Geometry: final body of the model. Coordinates: model frame, mm. Face numbers are marked on the shaded views. A direction names the side the tool comes from. Coordinates: 2 decimals unless noted, no trailing zeros. Write each loop counter-clockwise with the first axis right and the second up, starting at its lowest first coordinate (ties: lowest second). Pieces come first, ordered by that corner, then holes.
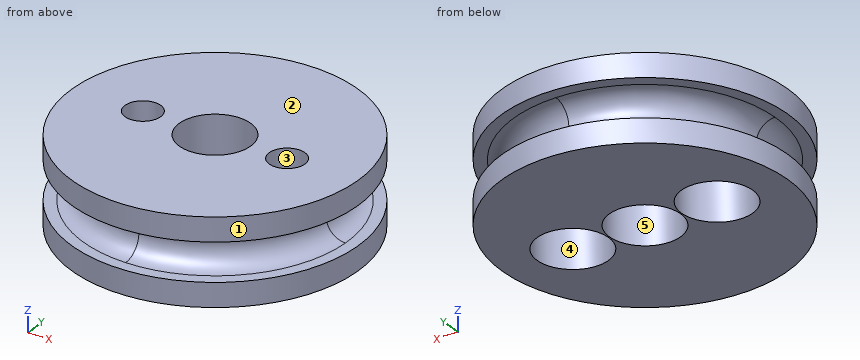
from build123d import *

# Parameters (mm, degrees)
SKETCH_1_R          = 12
EXTRUDE_1_DEPTH     = 2
SKETCH_2_R          = 11
EXTRUDE_2_DEPTH     = 3.2
SKETCH_3_R          = 12
EXTRUDE_3_DEPTH     = 2
SKETCH_4_R          = 3
CUT_EXTRUDE_1_DEPTH = 30
SKETCH_5_R          = 1.5
CUT_EXTRUDE_4_DEPTH = 19.434749795
SKETCH_3D_2_R       = 1.600287212
SKETCH_7_R          = 3
CUT_EXTRUDE_9_DEPTH = 4


with BuildPart() as part:
    # ｽｹｯﾁ1 → ﾎﾞｽ - 押し出し1 (new body)
    with BuildSketch(Plane.XY):
        Circle(SKETCH_1_R)
    extrude(amount=EXTRUDE_1_DEPTH)

    # ｽｹｯﾁ2 → ﾎﾞｽ - 押し出し2 (add)
    with BuildSketch(Plane.XY.offset(2)):
        Circle(SKETCH_2_R)
    extrude(amount=EXTRUDE_2_DEPTH)

    # ｽｹｯﾁ3 → ﾎﾞｽ - 押し出し3 (add)
    with BuildSketch(Plane.XY.offset(5.2)):
        Circle(SKETCH_3_R)
    extrude(amount=EXTRUDE_3_DEPTH)

    # ｽｹｯﾁ4 → ｶｯﾄ - 押し出し1 (cut)
    with BuildSketch(Plane(origin=(0, 0, 0), x_dir=(-1, 0, 0), z_dir=(0, 0, -1))):
        Circle(SKETCH_4_R)
    extrude(amount=-CUT_EXTRUDE_1_DEPTH, mode=Mode.SUBTRACT)

    # ｽｹｯﾁ5 → ｶｯﾄ - 押し出し4 (cut, through all)
    with BuildSketch(Plane(origin=(0, 0, 0), x_dir=(-1, 0, 0), z_dir=(0, 0, -1))):
        with Locations((-6.1, 0)):
            Circle(SKETCH_5_R)
        with Locations((6.1, 0)):
            Circle(SKETCH_5_R)
    extrude(amount=-CUT_EXTRUDE_4_DEPTH, mode=Mode.SUBTRACT)

    # ｶｯﾄ - ｽｲｰﾌﾟ2: sweep along a curve in space
    with BuildLine() as sweep_2_path:
        ThreePointArc((11, 0, 5.2), (7.778174593, 7.778174593, 5.2), (0, 11, 5.2))
        ThreePointArc((0, 11, 5.2), (-7.778174593, 7.778174593, 5.2), (-11, 0, 5.2))
        ThreePointArc((-11, 0, 5.2), (-7.778174593, -7.778174593, 5.2), (0, -11, 5.2))
        ThreePointArc((0, -11, 5.2), (7.778174593, -7.778174593, 5.2), (11, 0, 5.2))
    # Sketch 3D_2 → ｶｯﾄ - ｽｲｰﾌﾟ2 (sweep, cut)
    with BuildSketch(Plane(origin=(-11, 0, 5.2), x_dir=(0, 0, -1), z_dir=(0, -1, 0))):
        with Locations((1.600287212, 0)):
            Circle(SKETCH_3D_2_R)
    sweep(path=sweep_2_path.line, mode=Mode.SUBTRACT)

    # ｽｹｯﾁ7 → ｶｯﾄ - 押し出し9 (cut)
    with BuildSketch(Plane(origin=(0, 0, 0), x_dir=(-1, 0, 0), z_dir=(0, 0, -1))):
        with Locations((-6.1, 0)):
            Circle(SKETCH_7_R)
        with Locations((6.1, 0)):
            Circle(SKETCH_7_R)
    extrude(amount=-CUT_EXTRUDE_9_DEPTH, mode=Mode.SUBTRACT)


solid = part.part
Item 1: Section C-C, the plane z = 1.25. Output: boundary loops of the cut face in (x, y), plus the area to 3 significant figures.
Derived:
outline: circle Ø24 at (0, 0); hole circle Ø6 at (-6.1, 0); hole circle Ø6 at (0, 0); hole circle Ø6 at (6.1, 0)
area: 368 mm2
Item 2: Material intervals for probe 1 along Z at (x, y) = (-5.75, 10.5); probe 2 along X at (y, z) = (0.5, 3.5); probe 3 along X at (y, z) = (-0.5, 5.75), sorted ascending.
Derived:
probe 1: z = 0 to 2, 5.2 to 7.2
probe 2: x = -9.39 to -9.06, -3.14 to -2.96, 2.96 to 3.14, 9.06 to 9.39
probe 3: x = -11.99 to -7.51, -4.69 to -2.96, 2.96 to 4.69, 7.51 to 11.99
Item 3: Pull-direction query (Y, two-part tool) for the marked faces 1, 2 and 3; classes: released by +Y, released by -Y, zero draft, split by the parting line, or undercut.
Derived:
face 1: split by the parting line
face 2: zero draft
face 3: undercut
Item 4: Section A-A, the plane z = 6.5. Output: boundary loops of the cut face in (x, y).
Derived:
outline: circle Ø24 at (0, 0); hole circle Ø3 at (-6.1, 0); hole circle Ø6 at (0, 0); hole circle Ø3 at (6.1, 0)
Item 5: Section B-B, the plane y = 0.5. State how many separate pieces and enclosed holes the cut face has, plus the area to 3 significant figures.
Derived:
separate pieces: 4
enclosed holes: 0
area: 50.2 mm2
Item 6: Set-up query: the marked faces 4 and 5. Return all of +Z, -Z, +X, -X, +Y, -Y with unobstructed straight access to the full face (end or side cutting, diameter ignored); none if empty.
Derived:
face 4: -Z
face 5: +Z, -Z
Item 7: Pin query (flat end, axial travel): pin 1 (1 mm diameter, centred on x = -4, z = 6, fed in from +Y); pin 2 (2 mm diameter, centred on y = 3.5, z = 6, fed in from -X); pin 3 (4 mm diameter, centred on x = -6, z = 3.5, fed in from +Y); pin 4 (6.5 mm diameter, centred on x = -7, y = 0, fed in from -Z). Return the tip coordinate at first contact, or that it passes through.
Derived:
pin 1: stops at y = 11.48
pin 2: stops at x = -11.74
pin 3: stops at y = 11.05
pin 4: stops at z = 0
